Design review of the part shown in the three views and the two pictorial views. Dimensions are in mm from the part's minimum x, y and z. Round coordinates to 2 decimals unless told otherwise and drop trailing zeros. Order: outer loops, then holes, each group sorted by start corner. A loop starts at its lowest first (then second) coordinate and runs counter-clockwise, first axis right, second up. Notation, with made-up numbers: (1.25, 36) - (41.25, 36) arc R17 ccw to (41.25, 57) - close; hole circle Ø11 at (8, 60). An arc over 180 degrees is marked (long way). One line per question, with ' | ' between items. Start each with the question number.
Item 1: Add section C-C on x = 27. State the section outline as (y, z) points (1 decimal).
Item 2: Add section B-B on y = 1.5. State how many separate pieces and enclosed holes the cut face has, and give its area (3 significant figures).
Item 3: For L1, parallel to X at y = 1.4, z = 13 (1 decimal); L2, parallel to Z at x = 69, y = 0.7, list the stretches that pass through material, from the lowest coordinate up. Write a range as [from, to].
Item 4: Add section A-A on z = 20. State the section outline as (x, y) points (1 decimal), and give its area (3 significant figures).
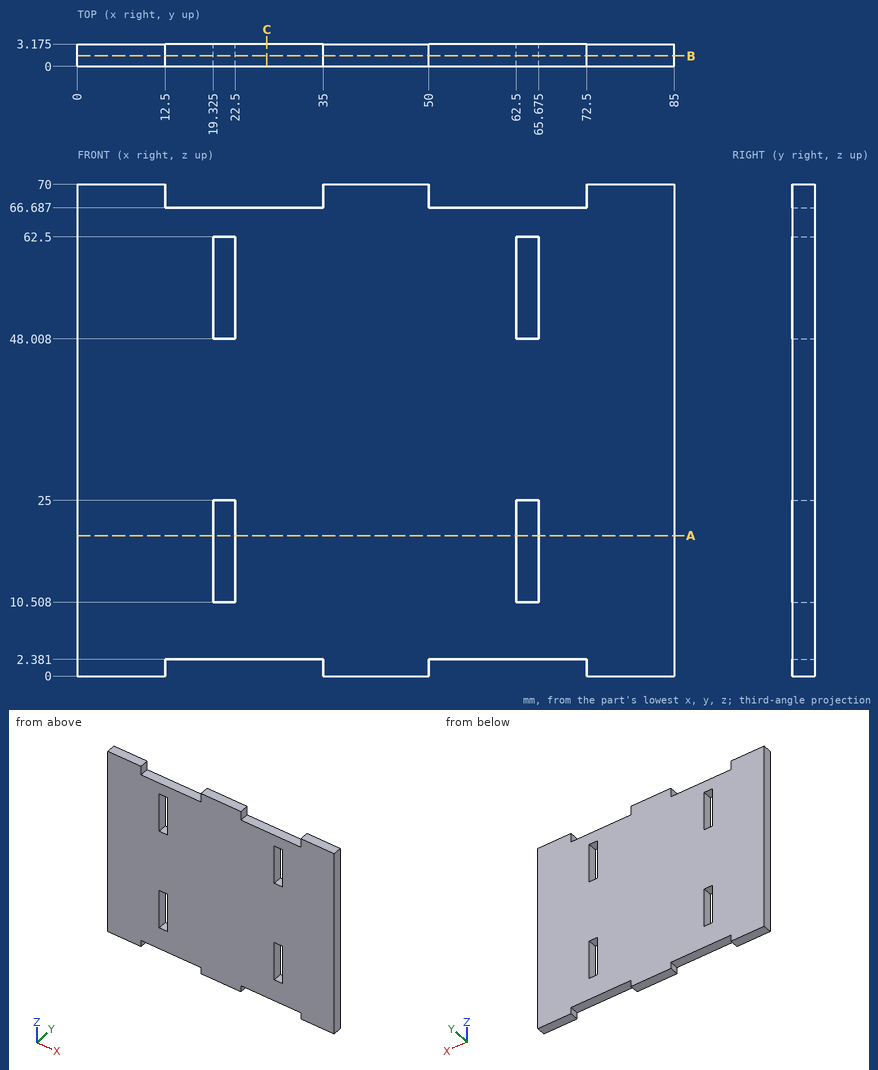
Determined:
1) outline: (0, 2.4) - (3.2, 2.4) - (3.2, 66.7) - (0, 66.7) - close
2) separate pieces: 1 | enclosed holes: 4 | area: 5,510 mm2
3) L1: [0, 19.3], [22.5, 62.5], [65.7, 85] | L2: [2.38, 66.69]
4) outline: (0, 0) - (19.3, 0) - (19.3, 3.2) - (0, 3.2) - close; (22.5, 0) - (62.5, 0) - (62.5, 3.2) - (22.5, 3.2) - close; (65.7, 0) - (85, 0) - (85, 3.2) - (65.7, 3.2) - close | area: 250 mm2
